```python
from build123d import *

# Parameters (mm, degrees)
SKETCH1_R               = 3.5
BOSS_EXTRUDE1_DEPTH     = 10
CUT_EXTRUDE1_DEPTH      = 3
CUT_EXTRUDE1_DEPTH_BACK = 3
CUT_EXTRUDE1_START      = -5
SKETCH2_R               = 3.5
SKETCH2_R_2             = 2.5


with BuildPart() as part:
    # Sketch1 → Boss-Extrude1 (new body)
    with BuildSketch(Plane.XY):
        Circle(SKETCH1_R)
    extrude(amount=BOSS_EXTRUDE1_DEPTH)

    # Sketch2 → Cut-Extrude1 (cut, two sides: drawn at the far end of the back side and taken through both)
    with BuildSketch(Plane.XY.offset(10).offset(CUT_EXTRUDE1_START - CUT_EXTRUDE1_DEPTH_BACK)):
        Circle(SKETCH2_R)
        Circle(SKETCH2_R_2, mode=Mode.SUBTRACT)
    extrude(amount=CUT_EXTRUDE1_DEPTH + CUT_EXTRUDE1_DEPTH_BACK, mode=Mode.SUBTRACT)


solid = part.part
```
Can you work these out from the model? Positions are in its coordinate system, mm. A direction names the side the tool comes from. Give positions to 0.01 mm unless a question says otherwise; leave off trailing zeros. Loops run counter-clockwise (first coordinate to the right, second up) from the corner with the lowest first, then second, coordinate; pieces in that order, holes last. Notation, with made-up numbers: M 17,18 L 74,18 A17 ccw 74,40 Z; hole C 84,6.5 d2. An arc over 180 degrees is marked long. Use CSV: the item, a comma, the result in double quotes. Start each with the question number.
1. On a 3-axis mill with a long thin cutter (end or side, diameter ignored), from which of +Z, -Z, +X, -X, +Y, -Y can I reach the whole of each face in a straight line? I mean faces 1 (the face through (3.233, -1.341, 8.986)), 2 (the face through (2, -2, 8)). Say none if no direction works.
2. Imagine slicing it at C-C, the plane y = 3. Write out the boundary of the cut face in (x, z).
3. If we mould it in two halves opening along Z, with no side actions, what happens to faces 3 (the face through (3.233, -1.341, 0.986)), 4 (the face through (0, 0, 0)), 5 (the face through (2, -2, 2)), 6 (the face through (0, 0, 10))? For each: released by +Z, released by -Z, zero draft, split by the parting line, or undercut.
4. If I drill on L1, parallel to Z at x = -2, y = 2.75; L2, parallel to Y at x = 2, z = 1.5; L3, parallel to Y at x = 1.5, z = 6.75, over which ranges is the centre line in solid material (lowest first)?
5. Imagine slicing it at A-A, the plane y = 0. Write out the boundary of the cut face in (x, z).
6. Imagine slicing it at D-D, the plane z = 2.25. Write out the boundary of the cut face in (x, y).
Response values:
1,face 1,"+Z, -Z"
1,face 2,"none"
2,outline,"M -1.8,0 L 1.8,0 L 1.8,2 L -1.8,2 Z; M -1.8,8 L 1.8,8 L 1.8,10 L -1.8,10 Z"
3,face 3,"zero draft"
3,face 4,"released by -Z"
3,face 5,"undercut"
3,face 6,"released by +Z"
4,L1,"0 to 2, 8 to 10"
4,L2,"-2.87 to 2.87"
4,L3,"-2 to 2"
5,outline,"M -3.5,0 L 3.5,0 L 3.5,2 L 2.5,2 L 2.5,8 L 3.5,8 L 3.5,10 L -3.5,10 L -3.5,8 L -2.5,8 L -2.5,2 L -3.5,2 Z"
6,outline,"C 0,0 d5"
